from build123d import *

# Parameters (mm, degrees)
EXTRUDE_1_DEPTH             = 13.5
CUT_EXTRUDE_1_DEPTH         = 9.5
SKETCH_3_W                  = 10
SKETCH_3_H                  = 13.5
EXTRUDE_2_DEPTH             = 11.133399735
SKETCH_4_W                  = 13.5
SKETCH_4_H                  = 46
EXTRUDE_3_DEPTH             = 20
CUT_EXTRUDE_2_DEPTH         = 9.5
CUT_EXTRUDE_3_DEPTH         = 55.538976888
SKETCH_7_W                  = 12.5
SKETCH_7_H                  = 13.5
HOLE_WIZARD_3_2_3_2_1_D     = 3.2
HOLE_WIZARD_3_2_3_2_1_DEPTH = 13.5
CHAMFER_1_SIZE              = 1.292893219
FILLET_1_R                  = 3.5
FILLET_2_R                  = 4
FILLET_3_R                  = 14


with BuildPart() as part:
    # 草图1 → 凸台-拉伸1 (new body)
    with BuildSketch(Plane.XY.offset(17)):
        with BuildLine():
            Line((13.5, -30), (19.5, -30))
            ThreePointArc((19.5, -30), (22.328427125, -28.828427125), (23.5, -26))
            Line((23.5, -26), (23.5, 18.866600265))
            Line((23.5, 18.866600265), (13.5, 18.866600265))
            ThreePointArc((13.5, 18.866600265), (12.334824944, 15.658155526), (9.382352941, 13.945070697))
            ThreePointArc((9.382352941, 13.945070697), (6.5, 10.5), (9.382352941, 7.054929303))
            ThreePointArc((9.382352941, 7.054929303), (12.334824944, 5.341844474), (13.5, 2.133399735))
            Line((13.5, 2.133399735), (13.5, -30))
        make_face()
    extrude(amount=-EXTRUDE_1_DEPTH)

    # 草图2 → 切除-拉伸1 (cut)
    with BuildSketch(Plane.XY.offset(17)):
        with BuildLine():
            Line((13.5, -20.343145751), (13.5, -30))
            Line((13.5, -30), (19.5, -30))
            ThreePointArc((19.5, -30), (20.366987609, -29.904911329), (21.192754868, -29.624166243))
            ThreePointArc((21.192754868, -29.624166243), (20.446463344, -29.435660891), (20.481374199, -28.666722312))
            ThreePointArc((20.481374199, -28.666722312), (20.822775499, -23.773082178), (16.166666667, -22.228763834))
            ThreePointArc((16.166666667, -22.228763834), (14.345299462, -21.976138912), (13.5, -20.343145751))
        make_face()
    extrude(amount=-CUT_EXTRUDE_1_DEPTH, mode=Mode.SUBTRACT)

    # 草图3 → 凸台-拉伸2 (add)
    with BuildSketch(Plane(origin=(0, 18.866600265, 0), x_dir=(-1, 0, 0), z_dir=(0, 1, 0))):
        with Locations((-18.5, 10.25)):
            Rectangle(SKETCH_3_W, SKETCH_3_H)
    extrude(amount=EXTRUDE_2_DEPTH)

    # 草图4 → 凸台-拉伸3 (add)
    with BuildSketch(Plane(origin=(23.5, 0, 0), x_dir=(0, 0, -1), z_dir=(1, 0, 0))):
        with Locations((-10.25, 7)):
            Rectangle(SKETCH_4_W, SKETCH_4_H)
    extrude(amount=EXTRUDE_3_DEPTH)

    # 草图5 → 切除-拉伸2 (cut)
    with BuildSketch(Plane.XY.offset(17)):
        with BuildLine():
            Line((23.156854249, 30), (13.5, 30))
            Line((13.5, 30), (13.5, 20.343145751))
            ThreePointArc((13.5, 20.343145751), (14.345299462, 21.976138912), (16.166666667, 22.228763834))
            ThreePointArc((16.166666667, 22.228763834), (20.328427125, 23.171572875), (21.271236166, 27.333333333))
            ThreePointArc((21.271236166, 27.333333333), (21.523861088, 29.154700538), (23.156854249, 30))
        make_face()
    extrude(amount=-CUT_EXTRUDE_2_DEPTH, mode=Mode.SUBTRACT)

    # 草图6 → 切除-拉伸3 (cut, through all)
    with BuildSketch(Plane(origin=(0, 0, 3.5), x_dir=(-1, 0, 0), z_dir=(0, 0, -1))):
        with BuildLine():
            Line((-33, -6.5), (-18, -6.5))
            Line((-18, -6.5), (-18, 0.5))
            ThreePointArc((-18, 0.5), (-25.5, -2), (-33, 0.5))
            Line((-33, 0.5), (-33, -6.5))
        make_face()
    extrude(amount=-CUT_EXTRUDE_3_DEPTH, mode=Mode.SUBTRACT)

    # 草图7 → 切除-旋转1 (revolve, cut)
    with BuildSketch(Plane(origin=(0, 10.5, 0), x_dir=(1, 0, 0), z_dir=(0, 1, 0))):
        with Locations((31.75, -10.25)):
            Rectangle(SKETCH_7_W, SKETCH_7_H)
    revolve(axis=Axis((25.5, 10.5, 3.5), (0, 0, 1)), mode=Mode.SUBTRACT)

    # Ø3.2 (3.2) 直径孔1
    with Locations(Plane(origin=(0, 0, 3.5), x_dir=(-1, 0, 0), z_dir=(0, 0, -1))):
        with Locations((-17.5, 26), (-17.5, -26)):
            Hole(HOLE_WIZARD_3_2_3_2_1_D / 2, depth=HOLE_WIZARD_3_2_3_2_1_DEPTH)

    # 倒角1
    chamfer_1_edges = [part.edges().sort_by_distance(p)[0] for p in [
        (33, -6.5, 10.25),
        (18, -6.5, 10.25),
    ]]
    chamfer(chamfer_1_edges, length=CHAMFER_1_SIZE)

    # 圆角1
    fillet_1_edges = [part.edges().sort_by_distance(p)[0] for p in [
        (33, 0.5, 10.25),
        (18, 0.5, 10.25),
    ]]
    fillet(fillet_1_edges, radius=FILLET_1_R)

    # 圆角2
    fillet_2_edges = [part.edges().sort_by_distance(p)[0] for p in [
        (13.5, -30, 5.5),
        (13.5, 30, 5.5),
        (23.5, -16, 10.25),
        (43.5, -16, 10.25),
    ]]
    fillet(fillet_2_edges, radius=FILLET_2_R)

    # 圆角3
    fillet_3_edges = [part.edges().sort_by_distance(p)[0] for p in [
        (43.5, 30, 10.25),
    ]]
    fillet(fillet_3_edges, radius=FILLET_3_R)


solid = part.part
Source: CAD feature listing. Evaluate the final solid. Frame: model axes, mm. A direction names the side the tool comes from. Give positions to 0.01 mm unless a question says otherwise; leave off trailing zeros. Write each loop counter-clockwise with the first axis right and the second up, starting at its lowest first coordinate (ties: lowest second). Pieces come first, ordered by that corner, then holes. Notation, with made-up numbers: (30.25, 16.5) - (41.25, 16.5) arc R21 cw to (41.25, 27.5) - close; hole circle Ø10 at (21, 88). An arc over 180 degrees is marked (long way). Write item = value, one per line. Start each with the question number.
Q1. Draft query along Y for faces 1 (the cylindrical face through (12.3, 5.38, 10.34)), 2 (the flat face through (13.5, 22, 7)), 3 (the cylindrical face through (20.284, 23.127, 12.317)). Return one class per face: +Y half, -Y half, draft (parallel to the pull), parting line (faces both ways), or undercut.
Q2. Cut plane C-C, the plane z = 6. Return loops of the section in (x, y).
Q3. Cut plane A-A, the plane x = 35.5. Return loops of the section in (y, z).
Q4. Cut plane B-B, the plane y = 10.5. Return loops of the section in (x, z), then the cut area to 3 significant figures.
Q5. Reachability of faces 4 (the flat face through (26, -6.5, 10)), 5 (the cylindrical face through (22.75, -28.33, 10.34)) from +Z, -Z, +X, -X, +Y, -Y: full face, straight path, thin tool, end or side. Return the list, or none.
Q6. Material intervals for probe 1 along Y at (x, z) = (17.5, 5.15); probe 2 along X at (y, z) = (10.5, 11.75); probe 3 along X at (y, z) = (-1, 15), sorted ascending.
Q7. Cut plane D-D, the plane z = 10. Return loops of the section in (x, y), then the cut area to 3 significant figures.
Q8. Pin query (flat end, axial travel): pin 1 Ø1.2 at (y, z) = (-2, 11) entering from -X; pin 2 Ø3.5 at (x, y) = (17.5, 26) entering from +Z; pin 3 Ø5 at (y, z) = (14.5, 12.5) entering from -X. Return the tip coordinate at first contact, or that it passes through.
Computed values:
q1.face_1 = -Y half
q1.face_2 = draft
q1.face_3 = undercut
q2.outline = (9.38, 7.05) arc R5 cw to (13.5, 2.13) - (13.5, -26) arc R4 ccw to (17.5, -30) - (19.5, -30) arc R4 ccw to (23.5, -26) - (23.5, -20) arc R4 cw to (27.5, -16) - (39.5, -16) arc R4 ccw to (43.5, -12) - (43.5, 16) arc R14 ccw to (29.5, 30) - (17.5, 30) arc R4 ccw to (13.5, 26) - (13.5, 18.87) arc R5 cw to (9.38, 13.95) arc R3.5 ccw to start; hole circle Ø3.2 at (17.5, -26); hole circle Ø3.2 at (17.5, 26); hole (16.91, 1.42) arc R3.5 cw to (18, -1.12) - (18, -5.21) - (19.29, -6.5) - (31.71, -6.5) - (33, -5.21) - (33, -1.12) arc R3.5 cw to (34.09, 1.42) arc R12.5 ccw (long way) to start
q3.outline = (-16, 3.5) - (3, 3.5) - (3, 17) - (-16, 17) - close; (18, 3.5) - (28.65, 3.5) - (28.65, 17) - (18, 17) - close
q4.outline = (6.5, 3.5) - (13, 3.5) - (13, 17) - (6.5, 17) - close; (38, 3.5) - (43.5, 3.5) - (43.5, 17) - (38, 17) - close
q4.area = 162 mm²
q5.face_4 = +Z, -Z
q5.face_5 = +Z, -Z, +X, -Y
q6.probe_1 = -30 to -27.6, -24.4 to 0.68, 20.1 to 24.4, 27.6 to 30
q6.probe_2 = 6.5 to 13, 38 to 43.5
q6.probe_3 = 13.5 to 18, 33 to 43.5
q7.outline = (9.38, 7.05) arc R5 cw to (13.5, 2.13) - (13.5, -20.34) arc R2 ccw to (16.17, -22.23) arc R4 cw to (20.48, -28.67) arc R0.61 ccw to (21.19, -29.62) arc R4 ccw to (23.5, -26) - (23.5, -20) arc R4 cw to (27.5, -16) - (39.5, -16) arc R4 ccw to (43.5, -12) - (43.5, 16) arc R14 ccw to (29.5, 30) - (23.16, 30) arc R2 ccw to (21.27, 27.33) arc R4 cw to (16.17, 22.23) arc R2 ccw to (13.5, 20.34) - (13.5, 18.87) arc R5 cw to (9.38, 13.95) arc R3.5 ccw to start; hole (16.91, 1.42) arc R3.5 cw to (18, -1.12) - (18, -5.21) - (19.29, -6.5) - (31.71, -6.5) - (33, -5.21) - (33, -1.12) arc R3.5 cw to (34.09, 1.42) arc R12.5 ccw (long way) to start
q7.area = 840 mm²
q8.pin_1 = 13.5
q8.pin_2 = 7.5
q8.pin_3 = 6.84
